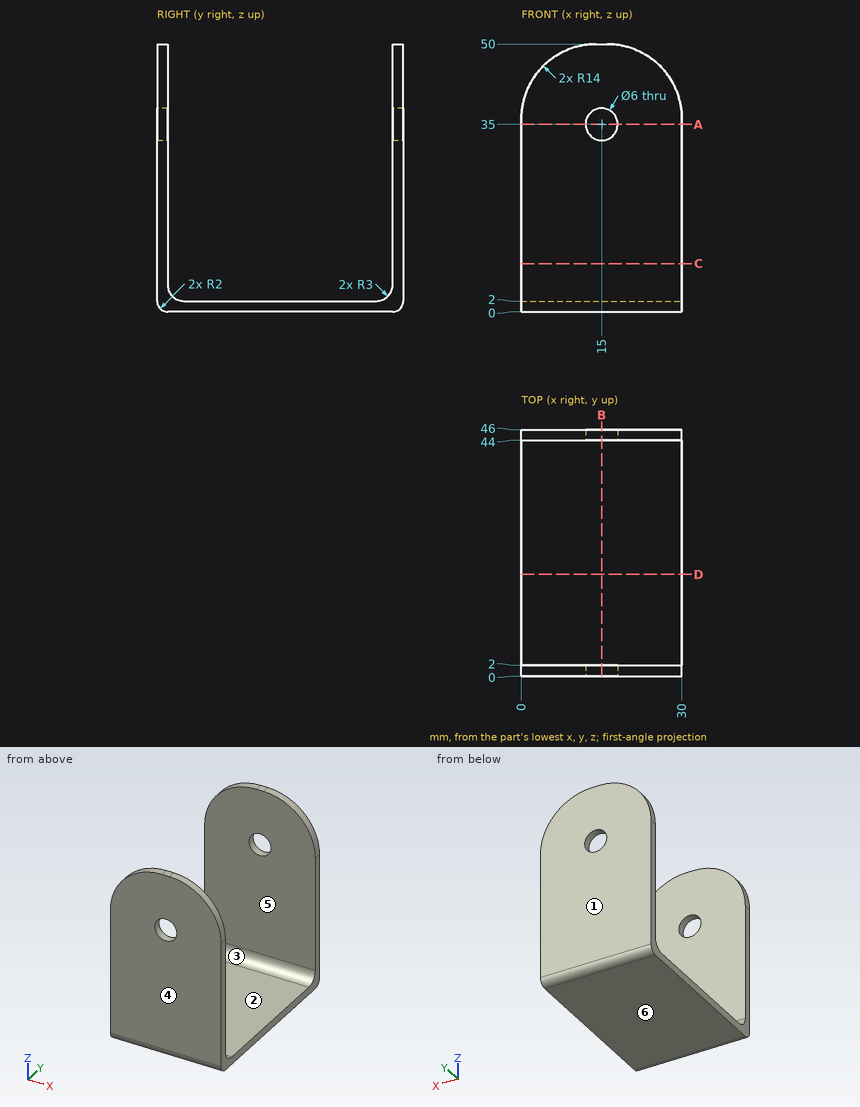
Can you work these out from the drawing? Everything is in mm from the part's minimum corner. A direction names the side the tool comes from. Coordinates: 2 decimals unless noted, no trailing zeros. Loops run counter-clockwise (first coordinate to the right, second up) from the corner with the lowest first, then second, coordinate; pieces in that order, holes last.
1. For P1, Ø15, axis at x = 9.5, y = 15, coming from the +Z side, with a flat end and sliding along its axis, tell me the tip position at first contact or that it passes through.
2. I need wall thicknesses on L1, parallel to Y at x = 4.5, z = 5; L2, parallel to X at y = 44.8, z = 35; L3, parallel to Z at x = 12, y = 8.5. Which ranges of each line are inside material? Lowest first, please.
3. Imagine slicing it at D-D, the plane y = 19. Please give me the cut outline in (x, z), and give its area (3 significant figures).
4. Imagine slicing it at C-C, the plane z = 9. Please give me the cut outline in (x, y).
5. Imagine slicing it at B-B, the plane x = 15. Please give me the cut outline in (y, z), and give its area (3 significant figures).
6. For the marked faces 5 and 6, which set-ups out of +Z, -Z, +X, -X, +Y, -Y let a thin tool reach every point of the face, with its end or its side?
7. If we mould it in two halves opening along Y, with no side actions, what happens to the marked faces 1, 2, 3 and 4? For each: pulls with the +Y half, pulls with the -Y half, needs draft (parallel to the pull), parting line crosses it, or undercut.
8. Imagine slicing it at A-A, the plane z = 35. Please give me the cut outline in (x, y).
Taken from the geometry:
1. P1: stops at z = 2
2. L1: y = 0 to 2, 44 to 46
2. L2: x = 0 to 12, 18 to 30
2. L3: z = 0 to 2
3. outline: (0, 0) - (30, 0) - (30, 2) - (0, 2) - close
3. area: 60.0 mm2
4. outline: (0, 0) - (30, 0) - (30, 2) - (0, 2) - close; (0, 44) - (30, 44) - (30, 46) - (0, 46) - close
5. outline: (0, 2) arc R2 ccw to (2, 0) - (44, 0) arc R2 ccw to (46, 2) - (46, 32) - (44, 32) - (44, 5) arc R3 cw to (41, 2) - (5, 2) arc R3 cw to (2, 5) - (2, 32) - (0, 32) - close; (0, 38) - (2, 38) - (2, 50) - (0, 50) - close; (44, 38) - (46, 38) - (46, 50) - (44, 50) - close
5. area: 262 mm2
6. face 5: +Z, +X, -X
6. face 6: -Z, +X, -X, +Y, -Y
7. face 1: pulls with the +Y half
7. face 2: undercut
7. face 3: undercut
7. face 4: pulls with the -Y half
8. outline: (0, 0) - (12, 0) - (12, 2) - (0, 2) - close; (0, 44) - (12, 44) - (12, 46) - (0, 46) - close; (18, 0) - (30, 0) - (30, 2) - (18, 2) - close; (18, 44) - (30, 44) - (30, 46) - (18, 46) - close
